Input: part model. Units: mm. Frame: model coordinates. Coordinates: 2 decimals unless noted, no trailing zeros. Write each loop counter-clockwise with the first axis right and the second up, starting at its lowest first coordinate (ties: lowest second). Pieces come first, ordered by that corner, then holes. Notation, with made-up numbers: (-7.75, -14.5) - (2.25, -14.5) arc R29 cw to (2.25, 9.5) - close; hole circle Ø5 at (-17.75, -5.75). An arc over 180 degrees is marked (long way). Use a Markdown table: item, result. Add a question column.
Q1. Section query A-A (y = -3). Return the cut outline in (x, z).
Q2. Pin query (flat end, axial travel): P1, Ø2, axis at x = -41, y = 75.5, coming from the -Z side; P2, Ø1.5, axis at x = -46.5, z = 2, coming from the +Y side. Return the tip coordinate at first contact, or that it passes through.
Q3. Section query B-B (z = 1.6). Give the number of separate pieces and of enclosed holes in the cut face, then the cut area to 3 significant figures.
Q4. Material intervals for probe 1 along X at (y, z) = (10.5, 1.05); probe 2 along Y at (x, z) = (-32.5, 2.3); probe 3 along Y at (x, z) = (-9, 0.85), sorted ascending. Write a range as from..to.
Q5. Mould query, pull axis X, two halves, no side actions, for faces 1 (the face through (10.68, -26.82, 1.48)), 2 (the face through (-10, 30, 3)), 3 (the face through (-9.222, 131.948, 1.479)). Classes: released by +X, released by -X, zero draft, split by the parting line, or undercut.
from build123d import *

# Parameters (mm, degrees)
F0_W     = 3.2
F0_H     = 12.24
F0_R     = 1.825
F0_R_2   = 2
F0_R_3   = 1.8
F0_R_4   = 1.65
F0_R_5   = 2.6
F1_DEPTH = 3


# Not quite as in the source:
# - ends of sketch curves that miss each other by under 0.0002 mm in the source are joined


with BuildPart() as f1:
    # F0 (on Top) → F1 (new body)
    with BuildSketch(Plane.XY):
        with BuildLine():
            Line((-69.459583357, 39.3533453141), (-69.459583357, -37.3673290014))
            Line((-69.459583357, -37.3673290014), (50.540416643, -37.3673290014))
            Line((50.540416643, -37.3673290014), (50.540416643, 39.3533036827))
            ThreePointArc((50.540416643, 39.3533036827), (50.404091241, 40.9988806108), (49.9988319578, 42.5995907516))
            add(Edge.make_bspline(
                [(6.5631451309, 127.1030604839), (13.1949586637, 122.5735143927), (26.4702997739, 107.0194370927), (36.3799750231, 82.2251008364), (45.1615562759, 56.6935268147), (49.9988319578, 42.5995907516)],
                knots=[0.1966855051, 0.1966855051, 0.1966855051, 0.1966855051, 0.4414351438, 0.6885909138, 0.9887974302, 0.9887974302, 0.9887974302, 0.9887974302], degree=3))
            ThreePointArc((6.5631451309, 127.1030604839), (-9.459583357, 131.9487932431), (-25.4823118448, 127.1030604839))
            add(Edge.make_bspline(
                [(-25.4823118448, 127.1030604839), (-32.1141253777, 122.5735143927), (-45.3894664879, 107.0194370927), (-55.2991588518, 82.2250580149), (-64.0807668858, 56.6933991917), (-68.9180648017, 42.5993980747)],
                knots=[0.1966855051, 0.1966855051, 0.1966855051, 0.1966855051, 0.4414351438, 0.6885909138, 0.9887987982, 0.9887987982, 0.9887987982, 0.9887987982], degree=3))
            ThreePointArc((-68.9180648017, 42.5993980747), (-69.323277955, 40.9988023559), (-69.459583357, 39.3533453141))
        make_face()
        with Locations((-46.859583357, -1.0729111145)):
            Rectangle(F0_W, F0_H, mode=Mode.SUBTRACT)
        with Locations((-27.459583357, -27.3673290014)):
            Circle(F0_R, mode=Mode.SUBTRACT)
        with Locations((-27.459583357, 9.0326709986)):
            Circle(F0_R, mode=Mode.SUBTRACT)
        with Locations((-40.759583357, 49.5270888855)):
            Circle(F0_R_2, mode=Mode.SUBTRACT)
        with Locations((8.940416643, -27.3673290014)):
            Circle(F0_R, mode=Mode.SUBTRACT)
        with Locations((8.940416643, 9.0326709986)):
            Circle(F0_R_3, mode=Mode.SUBTRACT)
        with Locations((27.940416643, -1.0729111145)):
            Rectangle(F0_W, F0_H, mode=Mode.SUBTRACT)
        with Locations((-40.759583357, 76.9270888855)):
            Circle(F0_R_2, mode=Mode.SUBTRACT)
        with Locations((-31.459583357, 103.8777989149)):
            Circle(F0_R_4, mode=Mode.SUBTRACT)
        with Locations((-9.459583357, 103.8777989149)):
            Circle(F0_R_4, mode=Mode.SUBTRACT)
        with Locations((-31.459583357, 114.8777989149)):
            Circle(F0_R_4, mode=Mode.SUBTRACT)
        with Locations((-9.459583357, 114.8777989149)):
            Circle(F0_R_4, mode=Mode.SUBTRACT)
        with Locations((-9.459583357, 123.8777989149)):
            Circle(F0_R_5, mode=Mode.SUBTRACT)
        with Locations((10.540416643, 81.9270888855)):
            Circle(F0_R_2, mode=Mode.SUBTRACT)
        with Locations((12.540416643, 103.8777989149)):
            Circle(F0_R_4, mode=Mode.SUBTRACT)
        with Locations((12.540416643, 114.8777989149)):
            Circle(F0_R_4, mode=Mode.SUBTRACT)
    extrude(amount=F1_DEPTH)


solid = f1.part
Values follow:
| question | item | result |
|---|---|---|
| 1 | outline | (-69.46, 0) - (-48.46, 0) - (-48.46, 3) - (-69.46, 3) - close; (-45.26, 0) - (26.34, 0) - (26.34, 3) - (-45.26, 3) - close; (29.54, 0) - (50.54, 0) - (50.54, 3) - (29.54, 3) - close |
| 2 | P1 | z = 0 |
| 2 | P2 | y = 103.45 |
| 3 | separate pieces | 1 |
| 3 | enclosed holes | 16 |
| 3 | area | 16,700 mm2 |
| 4 | probe 1 | -69.46..-28.54, -26.37..7.9, 9.98..50.54 |
| 4 | probe 2 | -37.37..102.6, 105.16..113.6, 116.16..121.17 |
| 4 | probe 3 | -37.37..102.29, 105.46..113.29, 116.46..121.32, 126.44..131.95 |
| 5 | face 1 | undercut |
| 5 | face 2 | zero draft |
| 5 | face 3 | split by the parting line |
